Input: part model. Units: mm. Frame: model coordinates. A direction names the side the tool comes from. Give positions to 0.01 mm unless a question says otherwise; leave off trailing zeros. Write each loop counter-clockwise with the first axis right and the second up, starting at its lowest first coordinate (ties: lowest second). Pieces come first, ordered by that corner, then holes.
Autodesk Inventor part; units mm, degrees
ref_plane "YZ Plane" through (0, 0, 0) normal (1, 0, 0) x (0, 1, 0)
ref_plane "XZ Plane" through (0, 0, 0) normal (0, 1, 0) x (-1, 0, 0)
ref_plane "XY Plane" through (0, 0, 0) normal (0, 0, 1) x (1, 0, 0)
sketch "Sketch1" plane through (0, 0, 0) normal (1, 0, 0) x (0, 1, 0)
  line L0 (0, 0) -> (30, 0)
  line L1 (30, 0) -> (0, 0)
  line L2 (0, 0) -> (0, -2.5)
  line L3 (0, -2.5) -> (30, -2.5)
  line L4 (30, -2.5) -> (30, 0)
  line L5 (30, -2.5) -> (27.5, -2.5)
  line L6 (27.5, -2.5) -> (27.5, -12.5)
  line L7 (27.5, -12.5) -> (30, -12.5)
  line L8 (30, -12.5) -> (30, -2.5)
  line L9 (0, -2.5) -> (2, -2.5)
  line L10 (2, -2.5) -> (2, -4.5)
  line L11 (2, -4.5) -> (0, -4.5)
  line L12 (0, -4.5) -> (0, -2.5)
  line L13 (0, -2.5) -> (-6, -2.5)
  line L14 (-6, -2.5) -> (-6, -4.5)
  line L15 (-6, -4.5) -> (0, -4.5)
  line L16 (0, -4.5) -> (0, -2.5)
  dimension "d0" = 30
  dimension "d1" = 2.5
  dimension "d2" = 2.5
  dimension "d3" = 10
  dimension "d4" = 2
  dimension "d5" = 2
  dimension "d6" = 6
extrude "Extrusion1" add sketch "Sketch1" along normal blind 50
sketch "Sketch2" plane through (0, 30, 0) normal (0, 1, 0) x (1, 0, 0)
  line L0 (50, 12.5) -> (50, 0)
  line L1 (50, 12.5) -> (45, 12.5)
  line L2 (45, 12.5) -> (45, 7.5)
  line L3 (45, 7.5) -> (50, 7.5)
  line L4 (50, 7.5) -> (50, 12.5)
  line L5 (45, 7.5) -> (35, 7.5)
  line L6 (0, 12.5) -> (50, 12.5)
  line L7 (0, 12.5) -> (5, 12.5)
  line L8 (5, 12.5) -> (5, 7.5)
  line L9 (5, 7.5) -> (0, 7.5)
  line L10 (0, 7.5) -> (0, 12.5)
  circle A0 centre (5, 7.5) radius 2
  circle A1 centre (35, 7.5) radius 2
  circle A2 centre (45, 7.5) radius 2
  line L11 (5, 7.5) -> (15, 7.5)
  circle A3 centre (15, 7.5) radius 2
  point P0 (0, 0)
  dimension "d9" = 5
  dimension "d10" = 5
  dimension "d11" = 10
  dimension "d12" = 5
  dimension "d13" = 5
  dimension "d14" = 4
  dimension "d15" = 4
  dimension "d16" = 4
  dimension "d19" = 10
  dimension "d20" = 4
extrude "Extrusion2" cut sketch "Sketch2" against normal blind 30 contours A1 | A3 | A2 L5 L3 | L3 L2 A2 | L2 L5 A2 | A0 L11 L8 | L8 L9 A0 | L11 A0 L9
sketch "Sketch3" plane through (0, 0, 0) normal (0, 0, 1) x (1, 0, 0)
  line L0 (0, -6) -> (0, 2)
  line L1 (0, -6) -> (5, -6)
  line L2 (5, -6) -> (5, 4)
  line L3 (5, 4) -> (0, 4)
  line L4 (0, 4) -> (0, -6)
  line L5 (45, -6) -> (40, -6)
  line L6 (40, -6) -> (40, 4)
  line L7 (40, 4) -> (45, 4)
  line L8 (45, 4) -> (45, -6)
  line L9 (50, -6) -> (50, 2)
  line L10 (50, -6) -> (45, -6)
  line L11 (45, -6) -> (45, 4)
  line L12 (45, 4) -> (50, 4)
  line L13 (50, 4) -> (50, -6)
  point P0 (0, 0)
  point P1 (0, 2)
  dimension "d21" = 5
  dimension "d22" = 10
  dimension "d23" = 5
  dimension "d24" = 10
extrude "Extrusion3" cut sketch "Sketch3" against normal blind 50 contours L0 L4 L3 L2 L1 | L8 L12 L13 L9 L10
sketch "Sketch4" plane through (0, 30, 0) normal (0, 0, 1) x (1, 0, 0)
  line L0 (0, 0) -> (0, -26)
  line L1 (0, -13) -> (50, -13)
  line L2 (50, -26) -> (50, -2.5)
  line L3 (0, -13) -> (10, -13)
  line L4 (10, -13) -> (20, -13)
  line L5 (20, -13) -> (30, -13)
  line L6 (30, -13) -> (40, -13)
  line L7 (40, -13) -> (50, -13)
  line L8 (7.5, -20.5) -> (12.5, -20.5)
  line L9 (12.5, -20.5) -> (12.5, -5.5)
  line L10 (12.5, -5.5) -> (7.5, -5.5)
  line L11 (7.5, -5.5) -> (7.5, -20.5)
  line L12 (7.5, -20.5) -> (12.5, -5.5) construction
  line L13 (12.5, -20.5) -> (7.5, -5.5) construction
  line L14 (17.5, -20.5) -> (22.5, -20.5)
  line L15 (22.5, -20.5) -> (22.5, -5.5)
  line L16 (22.5, -5.5) -> (17.5, -5.5)
  line L17 (17.5, -5.5) -> (17.5, -20.5)
  line L18 (17.5, -20.5) -> (22.5, -5.5) construction
  line L19 (22.5, -20.5) -> (17.5, -5.5) construction
  line L20 (27.5, -20.5) -> (32.5, -20.5)
  line L21 (32.5, -20.5) -> (32.5, -5.5)
  line L22 (32.5, -5.5) -> (27.5, -5.5)
  line L23 (27.5, -5.5) -> (27.5, -20.5)
  line L24 (27.5, -20.5) -> (32.5, -5.5) construction
  line L25 (32.5, -20.5) -> (27.5, -5.5) construction
  line L26 (37.5, -20.5) -> (42.5, -20.5)
  line L27 (42.5, -20.5) -> (42.5, -5.5)
  line L28 (42.5, -5.5) -> (37.5, -5.5)
  line L29 (37.5, -5.5) -> (37.5, -20.5)
  line L30 (37.5, -20.5) -> (42.5, -5.5) construction
  line L31 (42.5, -20.5) -> (37.5, -5.5) construction
  point P0 (0, -30)
  dimension "d27" = 10
  dimension "d28" = 10
  dimension "d29" = 10
  dimension "d30" = 10
  dimension "d31" = 10
  dimension "d32" = 5
  dimension "d33" = 15
  dimension "d34" = 5
  dimension "d35" = 15
  dimension "d36" = 5
  dimension "d37" = 15
  dimension "d38" = 5
  dimension "d39" = 15
extrude "Extrusion4" cut sketch "Sketch4" against normal blind 50
fillet "Fillet1" radius 2.5 16 edges at (7.5, 9.5, -1.25) (12.5, 9.5, -1.25) (7.5, 24.5, -1.25) (12.5, 24.5, -1.25) (17.5, 24.5, -1.25) (22.5, 24.5, -1.25) (17.5, 9.5, -1.25) (22.5, 9.5, -1.25) (27.5, 9.5, -1.25) (27.5, 24.5, -1.25) (32.5, 24.5, -1.25) (32.5, 9.5, -1.25) (37.5, 9.5, -1.25) (37.5, 24.5, -1.25) (42.5, 24.5, -1.25) (42.5, 9.5, -1.25)
fillet "Fillet2" radius 2.5 4 edges at (25, 30, 0) (25, 27.5, -2.5) (50, 4, -1.25) (0, 4, -1.25)
properties part number "lateral_panel_1"
Item 1: Pin query (flat end, axial travel): pin 1 (5 mm diameter, centred on x = 26.5, y = -4, fed in from +Z); pin 2 (5 mm diameter, centred on x = 27.5, y = 0.5, fed in from +Z); pin 3 (3.5 mm diameter, centred on y = 0, z = -2.5, fed in from +X); pin 4 (10 mm diameter, centred on x = 30, y = 14, fed in from -Z). Return the tip coordinate at first contact, or that it passes through.
Item 2: Section A-A (x = 15). Return loops of the section in (y, z), and give its area (3 significant figures).
Item 3: Set-up query: faces 5 (the flat face through (46, 4, -1)), 6 (the flat face through (25, 14, 0)), 7 (the cylindrical face through (21.787, 10.252, -1.268)). Return all of +Z, -Z, +X, -X, +Y, -Y with unobstructed straight access to the full face (end or side cutting, diameter ignored); none if empty.
Item 4: Section C-C (y = -3). Return loops of the section in (x, z), and give its area (3 significant figures).
Item 5: Section D-D (z = -6.5). Return loops of the section in (x, y), and give its area (3 significant figures).
Item 6: Section B-B (z = -8.75). Return loops of the section in (x, y), and give its area (3 significant figures).
Item 7: Ray query, line 1 (X direction, y = 28.25, z = -7.5); line 2 (X direction, y = 17.5, z = -1.5); line 3 (X direction, y = -1.5, z = -3.75). Return the intervals inside material, ascending.
Item 8: Mould query, pull axis X, two halves, no side actions, for faces 1 (the flat face through (25, 27.5, -9)), 2 (the flat face through (22.5, 17, -1)), 3 (the flat face through (50, 22, -2)), 4 (the cylindrical face through (43.526, 28.768, -8.852)). Classes: +X half, -X half, draft (parallel to the pull), parting line (faces both ways), or undercut.
Solved:
1. pin 1: stops at z = -2.5
1. pin 2: stops at z = 0
1. pin 3: stops at x = 45
1. pin 4: stops at z = -2.5
2. outline: (-6, -4.5) - (2, -4.5) - (2, -2.5) - (25, -2.5) arc R2.5 cw to (27.5, -5) - (27.5, -5.5) - (30, -5.5) - (30, -2.5) arc R2.5 ccw to (27.5, 0) - (0, 0) - (0, -2.5) - (-6, -2.5) - close; (27.5, -12.5) - (30, -12.5) - (30, -9.5) - (27.5, -9.5) - close
2. area: 106 mm2
3. face 5: +Z, -Z, +X, -Y
3. face 6: +Z, +X, -X, +Y, -Y
3. face 7: +Z, -Z
4. outline: (5, -4.5) - (45, -4.5) - (45, -2.5) - (5, -2.5) - close
4. area: 80.0 mm2
5. outline: (0, 27.5) - (3.27, 27.5) - (3.27, 30) - (0, 30) - close; (6.73, 27.5) - (13.27, 27.5) - (13.27, 30) - (6.73, 30) - close; (16.73, 27.5) - (33.27, 27.5) - (33.27, 30) - (16.73, 30) - close; (36.73, 27.5) - (43.27, 27.5) - (43.27, 30) - (36.73, 30) - close; (46.73, 27.5) - (50, 27.5) - (50, 30) - (46.73, 30) - close
5. area: 90.4 mm2
6. outline: (0, 27.5) - (3.44, 27.5) - (3.44, 30) - (0, 30) - close; (6.56, 27.5) - (13.44, 27.5) - (13.44, 30) - (6.56, 30) - close; (16.56, 27.5) - (33.44, 27.5) - (33.44, 30) - (16.56, 30) - close; (36.56, 27.5) - (43.44, 27.5) - (43.44, 30) - (36.56, 30) - close; (46.56, 27.5) - (50, 27.5) - (50, 30) - (46.56, 30) - close
6. area: 93.8 mm2
7. line 1: x = 0 to 3, 7 to 13, 17 to 33, 37 to 43, 47 to 50
7. line 2: x = 0 to 7.5, 12.5 to 17.5, 22.5 to 27.5, 32.5 to 37.5, 42.5 to 50
7. line 3: x = 5 to 45
8. face 1: draft
8. face 2: undercut
8. face 3: +X half
8. face 4: undercut
